CAD build for the part. Positions are in the model's coordinates, mm. A direction names the side the tool comes from. Give positions to 0.01 mm unless a question says otherwise; leave off trailing zeros. Loops run counter-clockwise (first coordinate to the right, second up) from the corner with the lowest first, then second, coordinate; pieces in that order, holes last. Notation, with made-up numbers: M 8,-20.75 L 31,-20.75 A20 ccw 31,-9.75 Z; hole C -1.75,67 d8. An arc over 180 degrees is marked long. One line per question, with ' | ' between items.
```python
from build123d import *

# Parameters (mm, degrees)
BOSS_EXTRUDE1_DEPTH     = 100
TENT_ANGLE_OUTSIDE_W    = 224.378
TENT_ANGLE_OUTSIDE_H    = 151.378
CUT_EXTRUDE1_DEPTH      = 139
CUT_EXTRUDE3_DEPTH      = 200
FILLET1_R               = 6
FILLET2_R               = 6
FEET_INSET_R            = 4.25
CUT_EXTRUDE4_DEPTH      = 0.6
FILLET3_R               = 2
CUT_EXTRUDE5_DEPTH      = 40
CUT_EXTRUDE5_DEPTH_BACK = 200


with BuildPart() as part:
    # base-outline → Boss-Extrude1 (new body)
    with BuildSketch(Plane(origin=(0, 0, 0), x_dir=(1, 0, 0), z_dir=(0, 1, 0))):
        Polygon((0, 10.82), (0, 0), (30, 0), (30, -3), (37, -3), (37, 0), (67, 0), (67, -3), (74, -3), (74, 0), (111, 0), (173, 0), (173, 139), (111, 139), (111, 142), (104, 142), (104, 139), (74, 139), (74, 142), (67, 142), (67, 139), (37, 139), (37, 142), (30, 142), (30, 139), (0, 139), (0, 128.18), (157, 128.18), (157, 10.82), align=None)
    extrude(amount=BOSS_EXTRUDE1_DEPTH)

    # tent-angle outside → Cut-Extrude1 (cut)
    with BuildSketch(Plane.XY):
        with Locations((86.5, 50)):
            Rectangle(TENT_ANGLE_OUTSIDE_W, TENT_ANGLE_OUTSIDE_H)
        Polygon((173, 57.723222932), (22.649180674, 3), (20.939079958, 7.698463104), (18.120002095, 6.672402674), (18.120002095, 0), (22.649180674, 0), (173, 0), align=None, mode=Mode.SUBTRACT)
    extrude(amount=-CUT_EXTRUDE1_DEPTH, mode=Mode.SUBTRACT)

    # middle-angle → Cut-Extrude3 (cut)
    with BuildSketch(Plane.XY):
        Polygon((161.698463104, 53.6097999), (173, 0), (173, 57.723222932), align=None)
    extrude(amount=-CUT_EXTRUDE3_DEPTH, mode=Mode.SUBTRACT)

    # Fillet1
    fillet1_edges = [part.edges().sort_by_distance(p)[0] for p in [
        (167.349231552, 26.80489995, 0),
    ]]
    fillet(fillet1_edges, radius=FILLET1_R)

    # Fillet2
    fillet2_edges = [part.edges().sort_by_distance(p)[0] for p in [
        (167.349231552, 26.80489995, -139),
    ]]
    fillet(fillet2_edges, radius=FILLET2_R)

    # feet-inset → Cut-Extrude4 (cut)
    with BuildSketch(Plane.XZ):
        with Locations(Location((45, -5.32, 0), (0, 0, 270))):
            Circle(FEET_INSET_R)
        with Locations(Location((165, -5.32, 0), (0, 0, 270))):
            Circle(FEET_INSET_R)
        with Locations(Location((165, -133.68, 0), (0, 0, 270))):
            Circle(FEET_INSET_R)
        with Locations(Location((45, -133.68, 0), (0, 0, 270))):
            Circle(FEET_INSET_R)
    extrude(amount=-CUT_EXTRUDE4_DEPTH, mode=Mode.SUBTRACT)

    # Fillet3
    fillet3_edges = [part.edges().sort_by_distance(p)[0] for p in [
        (104, 50, -142),
        (111, 50, -142),
        (74, 50, 3),
        (67, 50, 3),
        (37, 50, 3),
        (30, 50, 3),
        (30, 50, -142),
        (37, 50, -142),
        (67, 50, -142),
        (74, 50, -142),
    ]]
    fillet(fillet3_edges, radius=FILLET3_R)

    # keyboard-seat → Cut-Extrude5 (cut, two sides: drawn at the far end of the back side and taken through both)
    with BuildSketch(Plane.XY.offset(-CUT_EXTRUDE5_DEPTH_BACK)):
        Polygon((126.470388341, 150.398139841), (160.672402674, 56.428877763), (21.623120244, 5.819077862), (-12.578894088, 99.788339941), align=None)
    extrude(amount=CUT_EXTRUDE5_DEPTH + CUT_EXTRUDE5_DEPTH_BACK, mode=Mode.SUBTRACT)


solid = part.part
```
Item 1: Saw through at A-A on x = 45. Give the cut face in (y, z), and give its area (3 significant figures).
Conclusion:
outline: M 0,-139 L 11.14,-139 L 11.14,-128.18 L 0,-128.18 L 0,-129.43 L 0.6,-129.43 L 0.6,-137.93 L 0,-137.93 Z; M 0,-10.82 L 11.14,-10.82 L 11.14,0 L 0,0 L 0,-1.07 L 0.6,-1.07 L 0.6,-9.57 L 0,-9.57 Z | area: 231 mm²
Item 2: Mould opens along Z. For faces 1 (the flat face through (89, 12, -139)), 2 (the flat face through (120, 20, 0)), 3 (the flat face through (70, 22, 0)) say: pulls with the +Z half, pulls with the -Z half, needs draft (parallel to the pull), parting line crosses it, or undercut.
Conclusion:
face 1: pulls with the -Z half | face 2: pulls with the +Z half | face 3: undercut
Item 3: Drill centre lines: line 1 along Z through (x, y) = (150, 37.5); line 2 along Z through (x, y) = (108.5, 25.5); line 3 along X through (y, z) = (0.25, -5.32). Where is each one in solid material? Low to high. Write a range as [from, to].
Conclusion:
line 1: [-139, -128.18], [-10.82, 0] | line 2: [-142, -128.18], [-10.82, 0] | line 3: [18.12, 40.75], [49.25, 160.75], [169.25, 172.91]
Item 4: Saw through at C-C on x = 96.5. Give the cut face in (y, z).
Conclusion:
outline: M 0,-139 L 29.88,-139 L 29.88,-128.18 L 0,-128.18 Z; M 0,-10.82 L 29.88,-10.82 L 29.88,0 L 0,0 Z
Item 5: 3-axis set-ups, long thin cutter, end or side, ignore diameter. For faces 4 (the flat face through (139, 20, -139)), 5 (the flat face through (102, 20, -128.18)), 6 (the flat face through (21.806, 5.316, -133.514)), 7 (the flat face through (107, 36, -139)), 8 (the cylindrical face through (165.187, 0.296, -129.434)): which of +Z, -Z, +X, -X, +Y, -Y reach the whole face in a straight line?
Conclusion:
face 4: -Z, +X, +Y, -Y | face 5: -X, +Y, -Y | face 6: +Z, -Z, +Y | face 7: +Z, -X, +Y | face 8: -Y
Item 6: Saw through at B-B on z = -115.5. Give the cut face in (x, y).
Conclusion:
outline: M 157,0 L 173,0 L 161.7,53.61 L 157,51.9 Z
Item 7: Drop flat-ended pins along their axis: P1, Ø2.5, axis at x = 167, z = -134.5, coming from the -Y side; P2, Ø4, axis at y = 27.5, z = -54, coming from the -X side; P3, Ø0.5, axis at y = 3.5, z = -139.5, coming from the -X side; P4, Ø11, axis at x = 165, z = -133.68, coming from the -Y side. Give the stop position or say it passes through.
Conclusion:
P1: y = 0.6 | P2: x = 157 | P3: x = 30 | P4: y = 0
